```python
from build123d import *

# Parameters (mm, degrees)
F1_R = 15


with BuildPart() as f2:
    # F2: sweep along a path in F0
    with BuildLine(Plane.YZ) as f2_path:
        Line((0, 0), (0, 850))
        Line((0, 850), (200, 850))
        Line((200, 850), (200, 600))
        Line((200, 600), (600, 600))
        Line((600, 600), (600, 0))
    # F1 (on Top) → F2 (sweep)
    with BuildSketch(Plane.XY):
        Circle(F1_R)
    sweep(path=f2_path.line, transition=Transition.RIGHT)


solid = f2.part
```
Here's how the part is built. I have some questions about the finished solid (model axes, mm). A direction names the side the tool comes from. Give positions to 0.01 mm unless a question says otherwise; leave off trailing zeros. Order: outer loops, then holes, each group sorted by start corner. A loop starts at its lowest first (then second) coordinate and runs counter-clockwise, first axis right, second up. Notation, with made-up numbers: M -32,-18.75 L -15,-18.75 A15 ccw -15,10.25 Z; hole C 80.5,18 d3. An arc over 180 degrees is marked long. Use a Markdown table: item, result. Add a question column.
1. Suppose I cut it at C-C (y = 200). List the corners of the cut face in (x, z) for me, and give its area (3 significant figures).
2. Suppose I cut it at D-D (z = 850). List the corners of the cut face in (x, y) for me, and give its area (3 significant figures).
3. On a 3-axis mill with a long thin cutter (end or side, diameter ignored), from which of +Z, -Z, +X, -X, +Y, -Y can I reach the whole of each face in a straight line? I mean faces 4 (the flat face through (0, 0, 0)), 5 (the cylindrical face through (-14.985, 0.66, 438.555)), 6 (the cylindrical face through (-3.252, 101.61, 864.643)). Say none if no direction works.
4. For pin 1 Ø4 at (x, y) = (4, 147) entering from +Z; pin 2 Ø1.5 at (x, z) = (-4, 632.5) entering from -Y; pin 3 Ø3 at (x, y) = (2, 467) entering from +Z, each with a flat end and sliding along its axis, tell me the tip position at first contact or that it passes through.
5. Suppose I cut it at B-B (x = 0). List the corners of the cut face in (y, z) for me, and give its area (3 significant figures).
6. If we mould it in two halves opening along Y, with no side actions, what happens to faces 1 (the cylindrical face through (-3.252, 403.01, 614.643)), 2 (the cylindrical face through (-3.252, 214.643, 723.04)), 3 (the flat face through (0, 600, 0))? For each: +Y half, -Y half, draft (parallel to the pull), parting line (faces both ways), or undercut.
7. Suppose I cut it at A-A (z = 600). List the corners of the cut face in (x, y) for me, and give its area (3 significant figures).
8. I need wall thicknesses on probe 1 along Y at (x, z) = (-0.5, 287.5); probe 2 along Y at (x, z) = (-2.25, 195); probe 3 along Z at (x, y) = (0.75, 131). Which ranges of each line are inside material? Lowest first, please. Write a range as from..to.
Results list:
| question | item | result |
|---|---|---|
| 1 | outline | M -15,600 A15 ccw 15,600 L 15,850 A15 ccw -15,850 Z |
| 1 | area | 8,210 mm² |
| 2 | outline | M -15,0 A15 ccw 15,0 L 15,200 A15 ccw -15,200 Z |
| 2 | area | 6,710 mm² |
| 3 | face 4 | -Z, +X, -X, +Y, -Y |
| 3 | face 5 | -Z |
| 3 | face 6 | none |
| 4 | pin 1 | stops at z = 864.87 |
| 4 | pin 2 | stops at y = -14.64 |
| 4 | pin 3 | stops at z = 614.99 |
| 5 | outline | M -15,0 L 15,0 L 15,835 L 185,835 L 185,585 L 585,585 L 585,0 L 615,0 L 615,615 L 215,615 L 215,865 L -15,865 Z |
| 5 | area | 69,000 mm² |
| 6 | face 1 | undercut |
| 6 | face 2 | undercut |
| 6 | face 3 | draft |
| 7 | outline | C 0,0 d30; M -15,200 A15 ccw 15,200 L 15,600 A15 ccw -15,600 Z |
| 7 | area | 13,400 mm² |
| 8 | probe 1 | y = -14.99..14.99, 585.01..614.99 |
| 8 | probe 2 | y = -14.83..14.83, 585.17..614.83 |
| 8 | probe 3 | z = 835.02..864.98 |
